Input: dimensioned drawing with shaded views. Units: mm. Origin: part minimum x, y, z. Give positions to 0.01 mm unless a question says otherwise; leave off trailing zeros. Write each loop counter-clockwise with the first axis right and the second up, starting at its lowest first coordinate (ties: lowest second). Pieces come first, ordered by that corner, then holes. Notation, with made-up numbers: (-13, -2.5) - (23, -2.5) arc R21 cw to (23, 25.5) - close; hole circle Ø1 at (21.5, 9). An arc over 180 degrees is marked (long way). Answer as CSV lines item,"result".
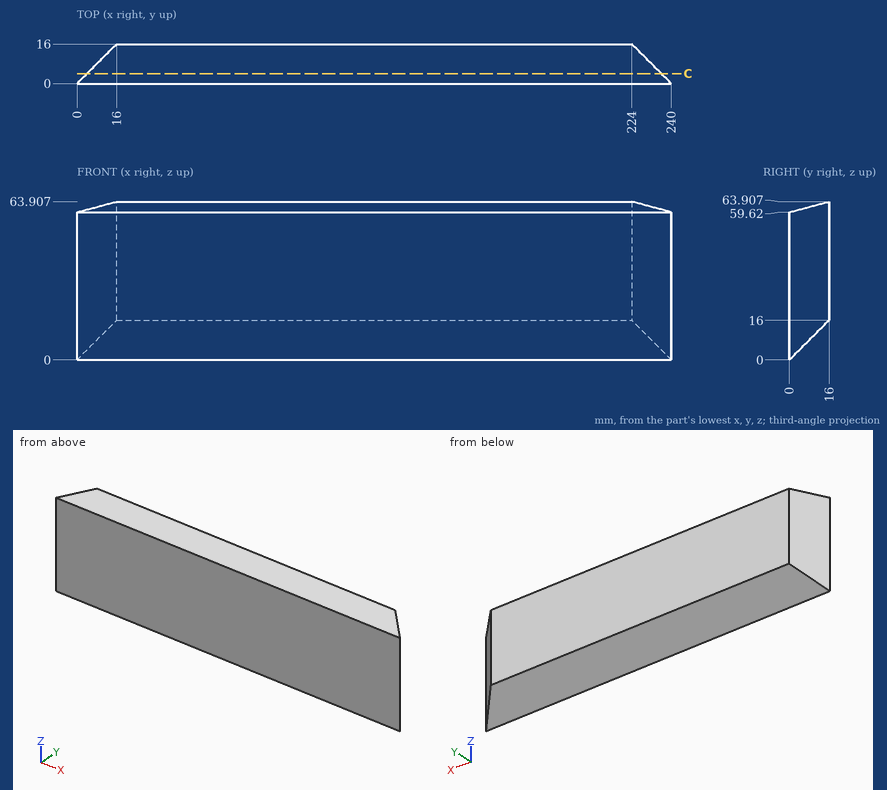
Item 1: Ray query, line 1 (Z direction, x = 66.5, y = 2.5); line 2 (Z direction, x = 219.5, y = 6.75); line 3 (Y direction, x = 13.5, z = 3.5). Return the intervals inside material, ascending. Write a range as from..to.
The answers:
line 1,"2.5..60.29"
line 2,"6.75..61.43"
line 3,"0..3.5"
Item 2: Contact query for flat-ended pins moving along their axis: pin 1 (2 mm diameter, centred on y = 1.5, z = 17, fed in from +X); pin 2 (5 mm diameter, centred on x = 144.5, y = 12, fed in from +Z) (1 decimal); pin 3 (3 mm diameter, centred on y = 7, z = 56, fed in from -X). Output: stop coordinate, or through.
The answers:
pin 1,"x = 239.5"
pin 2,"z = 63.5"
pin 3,"x = 5.5"
Item 3: Cut plane C-C on y = 4. Return the cut outline in (x, z), plus the area to 3 significant figures.
The answers:
outline,"(4, 4) - (236, 4) - (236, 60.69) - (4, 60.69) - close"
area,"13,200 mm²"
